Autodesk Inventor part; units mm, degrees
ref_plane "YZ Plane" through (0, 0, 0) normal (1, 0, 0) x (0, 1, 0)
ref_plane "XZ Plane" through (0, 0, 0) normal (0, 1, 0) x (-1, 0, 0)
ref_plane "XY Plane" through (0, 0, 0) normal (0, 0, 1) x (1, 0, 0)
sketch "Sketch1" plane through (0, 0, 0) normal (0, 0, 1) x (1, 0, 0)
  line L0 (-431.165, 0) -> (431.165, 0)
  line L1 (0, -416.56) -> (0, 99.06)
  line L2 (-307.975, 25.4) -> (307.975, 25.4)
  line L3 (-98.425, -342.9) -> (98.425, -342.9)
  line L4 (-307.975, 0) -> (-98.425, -342.9)
  line L5 (307.975, 0) -> (98.425, -342.9)
  line L6 (307.975, 0) -> (307.975, 25.4)
  line L7 (-307.975, 0) -> (-307.975, 25.4)
  point P0 (0, 0)
  point P1 (0, 25.4)
  point P2 (0, -342.9)
  point P3 (0, 25.4)
  dimension "d0" = 196.85
  dimension "d2" = 368.3
  dimension "d7" = 25.4
  dimension "d8" = 615.95
extrude "Extrusion1" add sketch "Sketch1" along normal mid plane 3.175
properties part number "electrical board back" material "ABS Plastic"
CAD build for the part. Positions are in the model's coordinates, mm. Round coordinates to 2 decimals unless told otherwise and drop trailing zeros. Loops run counter-clockwise (first coordinate to the right, second up) from the corner with the lowest first, then second, coordinate; pieces in that order, holes last.
(1) Cut at A-A (z = 0.15). Give the cut face in (x, y) (3 decimals).
(2) Wall check: line 1 along X through (y, z) = (-267.5, 1.15); line 2 along X through (y, z) = (-108.5, 0.3); line 3 along Y through (x, z) = (196.5, 1). Give the ranges that are in metal, low to high.
(3) Cut at B-B (y = -92.5). Give the cut face in (x, z), plus the area to 3 significant figures.
(4) Cut at C-C (x = -203). Give the cut face in (y, z).
(5) Drop a flat-ended pin along its axis: pin 1 (1.5 mm diameter, centred on y = -257.5, z = -1, fed in from -X). Give the stop position or say it passes through.
Findings below:
1. outline: (-307.975, 0) - (-98.425, -342.9) - (98.425, -342.9) - (307.975, 0) - (307.975, 25.4) - (-307.975, 25.4) - close
2. line 1: x = -144.5 to 144.5
2. line 2: x = -241.67 to 241.67
2. line 3: y = -182.41 to 25.4
3. outline: (-251.45, -1.59) - (251.45, -1.59) - (251.45, 1.59) - (-251.45, 1.59) - close
3. area: 1,600 mm2
4. outline: (-171.78, -1.59) - (25.4, -1.59) - (25.4, 1.59) - (-171.78, 1.59) - close
5. pin 1: stops at x = -151.07
